Can you work these out from the model? Positions are in its coordinate system, mm. A direction names the side the tool comes from. Give positions to 0.01 mm unless a question says otherwise; leave off trailing zeros. Write each loop counter-clockwise with the first axis right and the second up, starting at its lowest first coordinate (ties: lowest second). Pieces come first, ordered by that corner, then holes.
1. Suppose I cut it at B-B (x = 76). Please give me the cut outline in (y, z).
2. On a 3-axis mill with a long thin cutter (end or side, diameter ignored), from which of +Z, -Z, +X, -X, +Y, -Y can I reach the whole of each face in a straight line? I mean faces 1 (the flat face through (12.7, 55, 6)), 2 (the flat face through (110, 8.001, 10)), 3 (the flat face through (98, 10, 12.7)), 4 (the flat face through (223, 38, 4)), 5 (the flat face through (0, 55, 6)). Say none if no direction works.
3. Suppose I cut it at A-A (y = 55). Please give me the cut outline in (x, z), and give its area (3 significant figures).
4. I'm going to push flat-ended pins straight in: pin 1 (5 mm diameter, centred on x = 223.9, y = 71.97, fed in from -Z); pin 2 (6.5 mm diameter, centred on y = 71, z = 4.5, fed in from -X); pin 3 (0.8 mm diameter, centred on y = 7, z = 8.5, fed in from -X); pin 4 (0.5 mm diameter, centred on x = 67.5, y = 100.5, fed in from +Z). Where does each tip first touch, or does it pass through?
5. If I drill on probe 1 along Y at (x, z) = (136, 9.25); probe 2 along X at (y, z) = (91, 8.25); probe 3 along X at (y, z) = (73.5, 10.75), over which ranges is the centre line in solid material (lowest first)?
6. Thinking about a two-plate mould opening in Z: for faces 6 (the flat face through (110, 99.949, 10)), 7 (the flat face through (223, 74, 4)), 8 (the cylindrical face through (6.26, 73.65, 7.43)), which applies, pulls with the +Z half, pulls with the -Z half, needs draft (parallel to the pull), parting line crosses it, or undercut?
Autodesk Inventor part; units mm, degrees
ref_plane "YZ Plane" through (0, 0, 0) normal (1, 0, 0) x (0, 1, 0)
ref_plane "XZ Plane" through (0, 0, 0) normal (0, 1, 0) x (-1, 0, 0)
ref_plane "XY Plane" through (0, 0, 0) normal (0, 0, 1) x (1, 0, 0)
sketch "Sketch1" plane through (0, 0, 0) normal (0, 0, 1) x (1, 0, 0)
  line L0 (0, 0) -> (230.251, 0)
  line L1 (230.251, 0) -> (230.251, 107.95)
  line L2 (230.251, 107.95) -> (0, 107.95)
  line L3 (0, 107.95) -> (0, 0)
  line L4 (230.251, 107.95) -> (223.901, 107.95) construction
  line L5 (223.901, 107.95) -> (223.901, 101.6) construction
  line L6 (223.901, 101.6) -> (230.251, 101.6) construction
  line L7 (230.251, 101.6) -> (230.251, 107.95) construction
  line L8 (223.901, 101.6) -> (0, 101.6)
  line L9 (0, 101.6) -> (0, 100.076)
  line L10 (0, 100.076) -> (223.901, 100.076)
  line L11 (223.901, 100.076) -> (223.901, 101.6)
  line L12 (230.251, 0) -> (223.901, 0) construction
  line L13 (223.901, 0) -> (223.901, 35.9833) construction
  line L14 (223.901, 35.9833) -> (230.251, 35.9833) construction
  line L15 (230.251, 35.9833) -> (230.251, 0) construction
  circle A0 centre (223.901, 35.9833) radius 2
  circle A1 centre (223.901, 71.9667) radius 2
  line L16 (230.251, 53.975) -> (0, 53.975) construction
  line L17 (223.901, 6.35) -> (0, 6.35)
  line L18 (0, 7.874) -> (223.901, 7.874)
  line L19 (223.901, 7.874) -> (223.901, 6.35)
  dimension "length" = 230.251
  dimension "height" = 107.95
  dimension "d3" = 6.35
  dimension "d4" = 6.35
  dimension "d5" = 223.901
  dimension "d6" = 1.524
  dimension "spacing" = 35.9833
  dimension "d9" = 6.35
  dimension "TopScrewDiameter" = 4
  dimension "d13" = 35.9833
extrude "Generic Shape" add sketch "Sketch1" along normal blind 12.7
sketch "ScrewCapDiameter" plane through (0, 0, 0) normal (0, 0, -1) x (-1, 0, 0)
  circle A0 centre (-223.901, 71.9667) radius 2
  circle A1 centre (-223.901, 71.9667) radius 4
  circle A2 centre (-223.901, 35.9833) radius 2
  circle A3 centre (-223.901, 35.9833) radius 4
  point P0 (0, 0)
  dimension "d106" = 8
  dimension "d107" = 8
extrude "ScrewCapCountersink" cut sketch "ScrewCapDiameter" against normal blind 4
sketch "PcbNotchDimensions" plane through (0, 0, 12.7) normal (0, 0, 1) x (1, 0, 0)
  line L0 (230.251, 107.95) -> (0, 107.95) construction
  line L1 (230.251, 107.95) -> (223.901, 107.95) construction
  line L2 (223.901, 107.95) -> (223.901, 101.6) construction
  line L3 (223.901, 101.6) -> (230.251, 101.6) construction
  line L4 (230.251, 101.6) -> (230.251, 107.95) construction
  line L5 (223.901, 101.6) -> (0, 101.6)
  line L6 (0, 101.6) -> (0, 99.949)
  line L7 (0, 99.949) -> (223.901, 99.949)
  line L8 (223.901, 99.949) -> (223.901, 101.6)
  line L9 (230.251, 0) -> (230.251, 107.95) construction
  line L10 (230.251, 53.975) -> (0, 53.975) construction
  line L11 (0, 107.95) -> (0, 0) construction
  line L12 (223.901, 6.35) -> (0, 6.35)
  line L13 (0, 6.35) -> (0, 8.001)
  line L14 (0, 8.001) -> (223.901, 8.001)
  line L15 (223.901, 8.001) -> (223.901, 6.35)
  point P0 (230.251, 106.45)
  point P1 (0, 106.45)
  dimension "d21" = 6.35
  dimension "d22" = 6.35
  dimension "d23" = 223.901
  dimension "PcbThickness" = 1.651
extrude "PCB Notch" cut sketch "PcbNotchDimensions" against normal blind 6.35
sketch "UntappedScrewHoleDimensions" plane through (0, 0, 0) normal (-1, 0, 0) x (0, 0, 1)
  line L0 (0, 0) -> (6.35, 0) construction
  line L1 (6.35, 0) -> (6.35, 35.9833) construction
  line L2 (6.35, 35.9833) -> (0, 35.9833) construction
  line L3 (0, 35.9833) -> (0, 0) construction
  circle A0 centre (6.35, 35.9833) radius 2
  line L4 (0, 107.95) -> (6.35, 107.95) construction
  line L5 (6.35, 107.95) -> (6.35, 71.9667) construction
  line L6 (6.35, 71.9667) -> (0, 71.9667) construction
  line L7 (0, 71.9667) -> (0, 107.95) construction
  circle A1 centre (6.35, 71.9667) radius 2
  dimension "d33" = 6.35
  dimension "d34" = 35.9833
  dimension "ScrewDiameterUntapped" = 4
  dimension "d36" = 6.35
  dimension "d37" = 35.9833
  dimension "d38" = 4
extrude "UntappedScrewDepth" cut sketch "UntappedScrewHoleDimensions" against normal blind 12.7
thread "Thread10"
thread "Thread11"
sketch "Sketch18" plane through (0, 0, 0) normal (0, 0, -1) x (-1, 0, 0)
  line L0 (0, 0) -> (-12.7, 0) construction
  line L1 (-12.7, 0) -> (-12.7, 12.7) construction
  line L2 (-12.7, 12.7) -> (0, 12.7) construction
  line L3 (0, 12.7) -> (0, 0) construction
  line L4 (-12.7, 12.7) -> (-217.551, 12.7)
  line L5 (-217.551, 12.7) -> (-217.551, 95.25)
  line L6 (-217.551, 95.25) -> (-12.7, 95.25)
  line L7 (-12.7, 95.25) -> (-12.7, 12.7)
  dimension "bezel" = 12.7
  dimension "d156" = 12.7
  dimension "d157" = 204.851
  dimension "d158" = 82.55
extrude "Extrusion16" cut sketch "Sketch18" against normal blind 12.7
equation "\"d3\" = 0.5 * thickness"
equation "\"d4\" = 0.5 * thickness"
equation "\"d5\" = length - 0.5 * thickness"
equation "\"spacing\" = 0.333333 * height"
equation "\"d9\" = 0.5 * thickness"
equation "\"d13\" = spacing"
equation "\"d25\" = 0.5 * thickness"
equation "\"d33\" = 0.5 * thickness"
equation "\"d34\" = 0.333333 * height"
equation "\"d36\" = 0.5 * thickness"
equation "\"d37\" = 0.333333 * height"
equation "\"d38\" = ScrewDiameterUntapped"
equation "\"LcdThickness\" = 9.9"
properties part number "2020-04-11 CubeBaseSkeleton" material "PET Plastic"
Checks:
1. outline: (0, 0) - (12.7, 0) - (12.7, 12.7) - (8, 12.7) - (8, 6.35) - (6.35, 6.35) - (6.35, 12.7) - (0, 12.7) - close; (95.25, 0) - (107.95, 0) - (107.95, 12.7) - (101.6, 12.7) - (101.6, 6.35) - (99.95, 6.35) - (99.95, 12.7) - (95.25, 12.7) - close
2. face 1: +Z, -Z
2. face 2: +Z, -X
2. face 3: +Z, +X, -X, +Y, -Y
2. face 4: -Z
2. face 5: +Z, -Z, -X, +Y, -Y
3. outline: (0, 0) - (12.7, 0) - (12.7, 12.7) - (0, 12.7) - close; (217.55, 0) - (230.25, 0) - (230.25, 12.7) - (217.55, 12.7) - close
3. area: 323 mm2
4. pin 1: stops at z = 4
4. pin 2: stops at x = 0
4. pin 3: stops at x = 223.9
4. pin 4: stops at z = 6.35
5. probe 1: y = 0 to 6.35, 8 to 12.7, 95.25 to 99.95, 101.6 to 107.95
5. probe 2: x = 0 to 12.7, 217.55 to 230.25
5. probe 3: x = 0 to 12.7, 217.55 to 222.62, 225.19 to 230.25
6. face 6: needs draft
6. face 7: pulls with the -Z half
6. face 8: undercut
